from build123d import *

# Parameters (mm, degrees)
SKETCH1_W             = 6.4
SKETCH1_H             = 6.4
BOSS_EXTRUDE1_DEPTH   = 1
M3X0_5_TAPPED_HOLE1_D = 2.5
EDGE_FLANGE1_DEPTH    = 3
FILLET1_R             = 0.3


# Sheet-metal steps are written as plain solids
with BuildPart() as part:
    # Sketch1 → Boss-Extrude1 (new body)
    with BuildSketch(Plane(origin=(0, 0, 0), x_dir=(1, 0, 0), z_dir=(0, 1, 0))):
        Rectangle(SKETCH1_W, SKETCH1_H)
    extrude(amount=BOSS_EXTRUDE1_DEPTH)

    # M3x0.5 Tapped Hole1 (through all)
    with Locations(Plane(origin=(0, 1, 0), x_dir=(1, 0, 0), z_dir=(0, 1, 0))):
        with Locations((0, 0)):
            Hole(M3X0_5_TAPPED_HOLE1_D / 2)

    # Edge-Flange1 section (across the edge) → Edge-Flange1 (add)
    with BuildSketch(Plane(origin=(1.5, 0, 3.5), x_dir=(0, 0, -1), z_dir=(-1, 0, 0))):
        with BuildLine():
            Line((-1, 0.3), (-1, 3))
            Line((-1, 3), (0, 3))
            Line((0, 3), (0, 0.3))
            ThreePointArc((0, 0.3), (0.087867966, 0.087867966), (0.3, 0))
            Line((0.3, 0), (0.3, -1))
            ThreePointArc((0.3, -1), (-0.619238816, -0.619238816), (-1, 0.3))
        make_face()
    edge_flange1 = extrude(amount=EDGE_FLANGE1_DEPTH)

    # Mirror1: Edge-Flange1 across plane
    add(edge_flange1.mirror(Plane.XY))

    # Fillet1
    fillet1_edges = [part.edges().sort_by_distance(p)[0] for p in [
        (-3.2, 0.5, 3.2),
        (3.2, 0.5, 3.2),
        (3.2, 0.5, -3.2),
        (-3.2, 0.5, -3.2),
    ]]
    fillet(fillet1_edges, radius=FILLET1_R)


solid = part.part
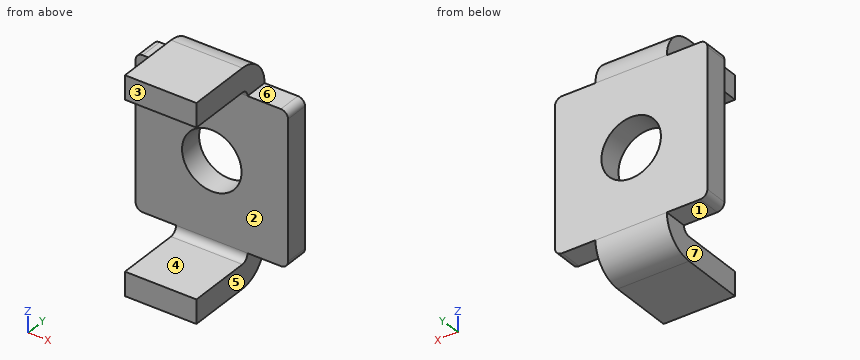
Input: part model. Units: mm. Frame: model coordinates. Face numbers are marked on the shaded views. A direction names the side the tool comes from. Coordinates: 2 decimals unless noted, no trailing zeros. Loops run counter-clockwise (first coordinate to the right, second up) from the corner with the lowest first, then second, coordinate; pieces in that order, holes last. Notation, with made-up numbers: (33.5, -10) - (77.5, -10) arc R23 ccw to (77.5, 1) - close; hole circle Ø9 at (62, 31). An arc over 180 degrees is marked (long way). Answer in a Markdown table with one row per item. Add a question column.
Item 1: Contact query for flat-ended pins moving along their axis: P1, Ø1.5, axis at y = -0.5, z = 0.5, coming from the -X side; P2, Ø0.8, axis at x = 2, y = 0.5, coming from the +Z side; P3, Ø1, axis at y = 0, z = 4, coming from the -X side; P4, Ø1, axis at y = 0, z = 4, coming from the +X side. Output: stop coordinate, or through.
Item 2: Line query: line 1 along Z through (x, y) = (0.5, -0.65); line 2 along Z through (x, y) = (0, 0.75); line 3 along Y through (x, z) = (-2.5, 3). Output: solid intervals per line, ascending. Write a range as [from, to].
Item 3: Section query B-B on x = 0. Return the cut outline in (y, z), then the cut area to 3 significant figures.
Item 4: Section query A-A on z = 0. Return the cut outline in (x, y), then the cut area to 3 significant figures.
Item 5: Section query C-C on y = -1. Return the cut outline in (x, z).
Item 6: Section query D-D on y = 0.65. Return the cut outline in (x, z).
Item 7: Access query for the marked faces 4, 5, 6 and 7. Directions: +Z, -Z, +X, -X, +Y, -Y. A direction counts if a zero-diameter tool reaches every point of the face in a straight line with its end or side. Return the directions, or none.
Item 8: Mould query, pull axis Z, two halves, no side actions, for the marked faces 1, 2 and 3. Classes: released by +Z, released by -Z, zero draft, split by the parting line, or undercut.
Recorded:
| question | item | result |
|---|---|---|
| 1 | P1 | x = -3.2 |
| 1 | P2 | z = 3.2 |
| 1 | P3 | x = -1.5 |
| 1 | P4 | x = 1.5 |
| 2 | line 1 | [-4.5, -3.5], [3.5, 4.5] |
| 2 | line 2 | [-3.97, -1.25], [1.25, 3.97] |
| 2 | line 3 | [0, 1] |
| 3 | outline | (-3, -4.5) - (-0.3, -4.5) arc R1.3 ccw to (1, -3.2) - (1, -1.25) - (0, -1.25) - (0, -3.2) arc R0.3 cw to (-0.3, -3.5) - (-3, -3.5) - close; (-3, 3.5) - (-0.3, 3.5) arc R0.3 cw to (0, 3.2) - (0, 1.25) - (1, 1.25) - (1, 3.2) arc R1.3 ccw to (-0.3, 4.5) - (-3, 4.5) - close |
| 3 | area | 11.8 mm^2 |
| 4 | outline | (-3.2, 0) - (-1.25, 0) - (-1.25, 1) - (-3.2, 1) - close; (1.25, 0) - (3.2, 0) - (3.2, 1) - (1.25, 1) - close |
| 4 | area | 3.90 mm^2 |
| 5 | outline | (-1.5, -4.5) - (1.5, -4.5) - (1.5, -3.5) - (-1.5, -3.5) - close; (-1.5, 3.5) - (1.5, 3.5) - (1.5, 4.5) - (-1.5, 4.5) - close |
| 6 | outline | (-3.2, -2.9) arc R0.3 ccw to (-2.9, -3.2) - (-1.5, -3.2) - (-1.5, -4.09) - (1.5, -4.09) - (1.5, -3.2) - (2.9, -3.2) arc R0.3 ccw to (3.2, -2.9) - (3.2, 2.9) arc R0.3 ccw to (2.9, 3.2) - (1.5, 3.2) - (1.5, 4.09) - (-1.5, 4.09) - (-1.5, 3.2) - (-2.9, 3.2) arc R0.3 ccw to (-3.2, 2.9) - close; hole circle Ø2.5 at (0, 0) |
| 7 | face 4 | +X, -X, -Y |
| 7 | face 5 | -Z, +X, +Y, -Y |
| 7 | face 6 | +Z, +X, +Y, -Y |
| 7 | face 7 | -Z, -X, +Y, -Y |
| 8 | face 1 | released by -Z |
| 8 | face 2 | undercut |
| 8 | face 3 | zero draft |
